Work out the finished part from the listing and answer in its coordinate system (mm). A direction names the side the tool comes from. Coordinates: 2 decimals unless noted, no trailing zeros. Loops run counter-clockwise (first coordinate to the right, second up) from the corner with the lowest first, then second, coordinate; pieces in that order, holes last.
```python
from build123d import *

# Parameters (mm, degrees)
F1_DEPTH = 31
F0_R     = 1.7
F0_R_2   = 5.2
F2_DEPTH = 6
F3_DEPTH = 4
F4_R     = 1.7
F5_DEPTH = 25


with BuildPart() as f1:
    # F0 (on Top) → F1 (new body)
    with BuildSketch(Plane.XY):
        with BuildLine():
            Line((12.6856816933, 0), (0, 0))
            Line((0, 0), (-12.6856816933, 0))
            Line((-12.6856816933, 0), (-22.3, 0))
            ThreePointArc((-22.3, 0), (-30, -7.7), (-37.7, 0))
            Line((-37.7, 0), (-45.7, 0))
            Line((-45.7, 0), (-57.7, 0))
            Line((-57.7, 0), (-57.7, -6))
            Line((-57.7, -6), (-44.5082735017, -6))
            ThreePointArc((-44.5082735017, -6), (-38.7261102445, -13.0516282509), (-30, -15.7))
            ThreePointArc((-30, -15.7), (-22.2253617447, -13.6398313773), (-16.4911140356, -8))
            Line((-16.4911140356, -8), (16.4911140356, -8))
            ThreePointArc((16.4911140356, -8), (22.2253617447, -13.6398313773), (30, -15.7))
            ThreePointArc((30, -15.7), (38.7261102445, -13.0516282509), (44.5082735017, -6))
            Line((44.5082735017, -6), (57.7, -6))
            Line((57.7, -6), (57.7, 0))
            Line((57.7, 0), (45.7, 0))
            Line((45.7, 0), (37.7, 0))
            ThreePointArc((37.7, 0), (30, -7.7), (22.3, 0))
            Line((22.3, 0), (12.6856816933, 0))
        make_face()
    extrude(amount=F1_DEPTH)

    # F0 (on Top) → F2 (join)
    with BuildSketch(Plane.XY):
        with BuildLine():
            Line((-12.6856816933, 0), (0, 0))
            Line((0, 0), (12.6856816933, 0))
            add(Edge.make_bspline(
                [(12.6856816933, 0), (12.3905999996, 2.441927908), (11.7188705001, 7.9681514968), (12.2103184435, 15.8432101865), (12.4767993137, 20.2387648954)],
                knots=[0, 0, 0, 0, 0.4418916914, 1, 1, 1, 1], degree=3))
            ThreePointArc((12.4767993137, 20.2387648954), (0, 33.5), (-12.4767993137, 20.2387648954))
            add(Edge.make_bspline(
                [(-12.6856816933, 0), (-12.3905999996, 2.441927908), (-11.7188705001, 7.9681514968), (-12.2103184435, 15.8432101865), (-12.4767993137, 20.2387648954)],
                knots=[0, 0, 0, 0, 0.4418916914, 1, 1, 1, 1], degree=3))
        make_face()
        with Locations((-8, 21)):
            Circle(F0_R, mode=Mode.SUBTRACT)
        with Locations((0, 13)):
            Circle(F0_R, mode=Mode.SUBTRACT)
        with Locations((0, 21)):
            Circle(F0_R_2, mode=Mode.SUBTRACT)
        with Locations((8, 21)):
            Circle(F0_R, mode=Mode.SUBTRACT)
        with Locations((0, 29)):
            Circle(F0_R, mode=Mode.SUBTRACT)
    extrude(amount=F2_DEPTH)

    # F0 (on Top) → F3 (join)
    with BuildSketch(Plane.XY):
        with BuildLine():
            ThreePointArc((-16.4911140356, -8), (-22.2253617447, -13.6398313773), (-30, -15.7))
            Line((-30, -15.7), (-30, -35.7866361737))
            Line((-30, -35.7866361737), (30, -35.7866361737))
            Line((30, -35.7866361737), (30, -15.7))
            ThreePointArc((30, -15.7), (22.2253617447, -13.6398313773), (16.4911140356, -8))
            Line((16.4911140356, -8), (-16.4911140356, -8))
        make_face()
    extrude(amount=F3_DEPTH)

    # F4 (on face) → F5 (cut)
    with BuildSketch(Plane.XZ.offset(8)):
        with Locations((-51.7, 19)):
            Circle(F4_R)
        with Locations((-8.3, 19)):
            Circle(F4_R)
        with Locations((8.3, 19)):
            Circle(F4_R)
        with Locations((51.7, 19)):
            Circle(F4_R)
    extrude(amount=-F5_DEPTH, mode=Mode.SUBTRACT)


solid = f1.part
```
1. A cutting plane is placed at D-D, the plane y = -30. Give the vertices of the cut face in (x, z).
2. A cutting plane is placed at A-A, the plane x = 0. Give the vertices of the cut face in (y, z).
3. A cutting plane is placed at C-C, the plane z = 22. Give the vertices of the cut face in (x, y).
4. For faces 1 (the flat face through (51, -6, 15)), 2 (the flat face through (0, -8, 17)), 3 (the flat face through (48, 0, 15)), determine the directions among +Z, -Z, +X, -X, +Y, -Y from which every point of the face is accessible in a straight line to the end or side of a thin tool.
5. Each of these flat-tipped pins is pushed along its axis until it touches: P1, Ø2, axis at x = -3.5, y = -20.5, coming from the +Z side; P2, Ø1, axis at x = -24.5, z = 5, coming from the -Y side; P3, Ø8, axis at x = -8, z = 20.5, coming from the -Y side; P4, Ø2.5, axis at x = 8.3, z = 19, coming from the -Y side. Where does it stop, or does it pass through?
6. A cutting plane is placed at B-B, the plane x = 51.7. Give the vertices of the cut face in (y, z).
7. Straight lines are drawn through the part: probe 1 along Y at (x, z) = (0, 2.8); probe 2 along Z at (x, y) = (51.7, -2.6); probe 3 along X at (y, z) = (-10, 29.5). For each, find the intervals that lie inside material, in ascending order.
8. Determine the mould class of faces 4 (the cylindrical face through (-0.221, 30.686, 2.958)), 5 (the cylindrical face through (9.92, -4.06, 19.51)), 6 (the cylindrical face through (-8.221, 22.686, 2.958)), 7 (the flat face through (-48, 0, 15)) for opening direction Y: released by +Y, released by -Y, zero draft, split by the parting line, or undercut.
Answers below:
1. outline: (-30, 0) - (30, 0) - (30, 4) - (-30, 4) - close
2. outline: (-35.79, 0) - (11.3, 0) - (11.3, 6) - (0, 6) - (0, 31) - (-8, 31) - (-8, 4) - (-35.79, 4) - close; (14.7, 0) - (15.8, 0) - (15.8, 6) - (14.7, 6) - close; (26.2, 0) - (27.3, 0) - (27.3, 6) - (26.2, 6) - close; (30.7, 0) - (33.5, 0) - (33.5, 6) - (30.7, 6) - close
3. outline: (-57.7, -6) - (-44.51, -6) arc R15.7 ccw to (-16.49, -8) - (16.49, -8) arc R15.7 ccw to (44.51, -6) - (57.7, -6) - (57.7, 0) - (37.7, 0) arc R7.7 cw to (22.3, 0) - (-22.3, 0) arc R7.7 cw to (-37.7, 0) - (-57.7, 0) - close
4. face 1: +Z, -Z, +X, -Y
4. face 2: +Z, -Y
4. face 3: +Z, -Z, +X, +Y
5. P1: stops at z = 4
5. P2: stops at y = -14.88
5. P3: stops at y = -8
5. P4: passes through
6. outline: (-6, 0) - (0, 0) - (0, 17.3) - (-6, 17.3) - close; (-6, 20.7) - (0, 20.7) - (0, 31) - (-6, 31) - close
7. probe 1: y = -35.79 to 11.3, 14.7 to 15.8, 26.2 to 27.3, 30.7 to 33.5
7. probe 2: z = 0 to 17.3, 20.7 to 31
7. probe 3: x = -42.1 to -17.9, 17.9 to 42.1
8. face 4: undercut
8. face 5: zero draft
8. face 6: undercut
8. face 7: released by +Y
